Build history of the part. All positions in model axes, mm. Face numbers are marked on the shaded views. Round coordinates to 2 decimals unless told otherwise and drop trailing zeros. Loops run counter-clockwise (first coordinate to the right, second up) from the corner with the lowest first, then second, coordinate; pieces in that order, holes last.
Autodesk Inventor part; units mm, degrees
ref_plane "YZ Plane" through (0, 0, 0) normal (1, 0, 0) x (0, 1, 0)
ref_plane "XZ Plane" through (0, 0, 0) normal (0, 1, 0) x (-1, 0, 0)
ref_plane "XY Plane" through (0, 0, 0) normal (0, 0, 1) x (1, 0, 0)
sketch "Sketch1" plane through (0, 0, 0) normal (1, 0, 0) x (0, 1, 0)
  circle A0 centre (0, 0) radius 4.572
  circle A1 centre (0, 0) radius 8.382
  dimension "d0" = 9.144
  dimension "d1" = 3.81
extrude "Extrusion1" add sketch "Sketch1" along normal blind 19.812
sketch "Sketch2" plane through (0, 0, 0) normal (-1, 0, 0) x (0, 0, 1)
  circle A0 centre (0, 0) radius 8.382
  circle A1 centre (0, 0) radius 7.747
  circle A2 centre (0, 0) radius 8.382
  dimension "d42" = 0
extrude "Extrusion2" add sketch "Sketch2" along normal blind 2.54 contours A0 | A1
sketch "Sketch3" plane through (-2.54, 0, 0) normal (-1, 0, 0) x (0, 0, 1)
  line L0 (19.05, 48.5955) -> (-19.05, 48.5955)
  circle A0 centre (0, 0) radius 8.382
  line L1 (8.382, 0) -> (19.05, 48.5955)
  line L2 (-8.382, 0) -> (-19.05, 48.5955)
  arc A1 (8.382, 0) -> (-8.382, 0) centre (0, 0) ccw
  line L3 (-14.3129, 44.7855) -> (14.3129, 44.7855)
  line L4 (14.3129, 44.7855) -> (6.7152, 10.176)
  arc A2 (6.7152, 10.176) -> (-6.7152, 10.176) centre (0, 0) ccw
  line L5 (-6.7152, 10.176) -> (-14.3129, 44.7855)
  dimension "d6" = 38.1
  dimension "d7" = 19.05
  dimension "d8" = 3.81
extrude "Extrusion3" add sketch "Sketch3" against normal blind 6.35 contours L1 A0 L2 L0
sketch "Sketch6" plane through (-2.54, 44.7855, -14.3129) normal (0, -1, 0) x (1, 0, 0)
  line L0 (6.35, 32.4159) -> (26.9875, 32.4159)
  line L1 (13.4874, 32.4159) -> (13.4874, 26.0989)
  line L2 (26.9875, 32.4159) -> (26.9875, -3.9117)
  point P0 (2.54, 14.3129)
  dimension "d20" = 13.5001
sketch "Sketch10" plane through (0, 0, 0) normal (1, 0, 0) x (0, 0, -1)
  circle A0 centre (0, 0) radius 1.4542
  line L0 (-4.572, 1.4542) -> (4.572, 1.4542)
  line L1 (4.572, 1.4542) -> (4.572, -1.4542)
  line L2 (4.572, -1.4542) -> (-4.572, -1.4542)
  line L3 (-4.572, -1.4542) -> (-4.572, 1.4542)
  circle A1 centre (0, 0) radius 4.572
  dimension "d43" = 0
  dimension "d44" = 0
extrude "Extrusion7" cut sketch "Sketch10" against normal blind 22.225 contours A0 | A0 L0 A1 L2 | A0 L2 A1 L0 | A1 L3 L0 | L0 L1 A1 | A1 L1 L2 | L2 L3 A1
sketch "Sketch13" plane through (-2.54, 48.5955, 19.05) normal (0, 1, 0) x (1, 0, 0)
  line L0 (4.6355, 36.83) -> (1.7145, 36.83)
  line L1 (1.7145, 36.83) -> (1.7145, 33.909)
  line L2 (1.7145, 33.909) -> (4.6355, 33.909)
  line L3 (4.6355, 33.909) -> (4.6355, 36.83)
  line L4 (6.35, 38.1) -> (6.35, 0)
  line L5 (0, 38.1) -> (6.35, 38.1)
  line L6 (4.6228, 4.191) -> (1.7018, 4.191)
  line L7 (1.7018, 4.191) -> (1.7018, 1.27)
  line L8 (1.7018, 1.27) -> (4.6228, 1.27)
  line L9 (4.6228, 1.27) -> (4.6228, 4.191)
  line L10 (0, 0) -> (6.35, 0)
  line L11 (0, 0) -> (0, 38.1)
  line L12 (0, 0) -> (6.35, 0)
  line L13 (6.35, 38.1) -> (6.35, 0)
  line L14 (0, 38.1) -> (6.35, 38.1)
  point P0 (2.54, 19.05)
  dimension "d32" = 2.921
  dimension "d33" = 2.921
  dimension "d34" = 1.7145
  dimension "d35" = 1.27
  dimension "d36" = 2.921
  dimension "d37" = 2.921
  dimension "d38" = 1.7272
  dimension "d39" = 1.27
extrude "Extrusion9" add sketch "Sketch13" along normal blind 3.81 contours L3 L2 L1 L0 | L4 L10 L11 L5 | L9 L8 L7 L6
sketch "Sketch14" plane through (0, 0, 0) normal (-1, 0, 0) x (0, 0, 1)
  arc A0 (4.3346, -1.4542) -> (4.572, 0) centre (0, 0) ccw
  line L0 (4.3346, -1.4542) -> (4.572, -1.4542)
  line L1 (4.572, -1.4542) -> (4.572, 0)
  arc A1 (4.572, 0) -> (4.3346, 1.4542) centre (0, 0) ccw
  line L2 (4.572, 0) -> (4.572, 1.4542)
  line L3 (4.572, 1.4542) -> (4.3346, 1.4542)
  arc A2 (-4.572, 0) -> (-4.3346, -1.4542) centre (0, 0) ccw
  line L4 (-4.572, 0) -> (-4.572, -1.4542)
  line L5 (-4.572, -1.4542) -> (-4.3346, -1.4542)
  arc A3 (-4.3346, 1.4542) -> (-4.572, 0) centre (0, 0) ccw
  line L6 (-4.3346, 1.4542) -> (-4.572, 1.4542)
  line L7 (-4.572, 1.4542) -> (-4.572, 0)
extrude "Extrusion10" add sketch "Sketch14" along normal blind 2.54
sketch "Sketch15" plane through (-2.54, 0, 0) normal (-1, 0, 0) x (0, 0, 1)
  circle A0 centre (0, 0) radius 41.275
  circle A1 centre (0, 0) radius 44.45
  dimension "d47" = 82.55
  dimension "d48" = 88.9
extrude "Extrusion11" add sketch "Sketch15" against normal blind 2.54
sketch "Sketch16" plane through (0, 0, 0) normal (1, 0, 0) x (0, 0, -1)
  circle A0 centre (0, 0) radius 44.45
  circle A1 centre (0, 0) radius 41.275
  dimension "d51" = 82.55
extrude "Extrusion12" add sketch "Sketch16" along normal blind 31.75
sketch "Sketch19" plane through (-2.54, 0, 0) normal (-1, 0, 0) x (0, 0, 1)
  line L0 (4.3346, 1.4542) -> (-4.3346, 1.4542)
  arc A0 (-16.671, 37.7585) -> (16.671, 37.7585) centre (0, 0) ccw
  line L1 (-4.3346, 1.4542) -> (-41.2494, 1.4542)
  line L2 (4.3346, 1.4542) -> (41.2494, 1.4542)
  circle A1 centre (0, 0) radius 8.382
  line L3 (-4.3346, -1.4542) -> (4.3346, -1.4542)
  line L4 (4.3346, 1.4542) -> (-4.3346, 1.4542)
  line L5 (-41.2494, -1.4542) -> (41.2494, -1.4542)
extrude "Extrusion14" add sketch "Sketch19" against normal blind 6.35 contours L2 A1 L5 L3 L1 L0 | L2 A0 L5 A1 | A1 L5 A0 L1
sketch "Sketch20" plane through (3.81, 0, 0) normal (1, 0, 0) x (0, 0, -1)
  arc A0 (4.3346, -1.4542) -> (4.3346, 1.4542) centre (0, 0) ccw
  line L0 (4.3346, 1.4542) -> (-4.3346, 1.4542)
  arc A1 (-4.3346, 1.4542) -> (-4.3346, -1.4542) centre (0, 0) ccw
  line L1 (-4.3346, -1.4542) -> (4.3346, -1.4542)
extrude "Extrusion15" cut sketch "Sketch20" against normal blind 6.35
sketch "Sketch21" plane through (-2.54, 0, 0) normal (-1, 0, 0) x (0, 0, 1)
  arc A0 (-8.2549, -1.4542) -> (8.2549, -1.4542) centre (0, 0) ccw
  line L0 (1.8492, -8.1755) -> (1.8492, -41.2336)
  arc A1 (-41.2494, -1.4542) -> (41.2494, -1.4542) centre (0, 0) ccw
  line L1 (-1.8492, -41.2336) -> (-1.8492, -8.1755)
  arc A2 (-1.8492, -8.1755) -> (1.8492, -8.1755) centre (0, 0) ccw
  arc A3 (-1.8492, -41.2336) -> (1.8492, -41.2336) centre (0, 0) ccw
extrude "Extrusion16" add sketch "Sketch21" against normal blind 6.35
sketch "Sketch23" plane through (3.81, 0, 0) normal (1, 0, 0) x (0, 0, -1)
  line L0 (19.05, 52.4055) -> (-19.05, 52.4055)
  line L1 (-19.05, 48.5955) -> (-19.05, 52.4055)
  line L2 (19.05, 52.4055) -> (-19.05, 52.4055)
  line L3 (-19.05, 52.4055) -> (-19.05, 48.5955)
  line L4 (-19.05, 48.5955) -> (19.05, 48.5955)
  line L5 (19.05, 48.5955) -> (19.05, 52.4055)
  point P0 (0, 0)
extrude "Extrusion17" add sketch "Sketch23" along normal blind 19.05
properties part number "BasicThrustMotorHousing"
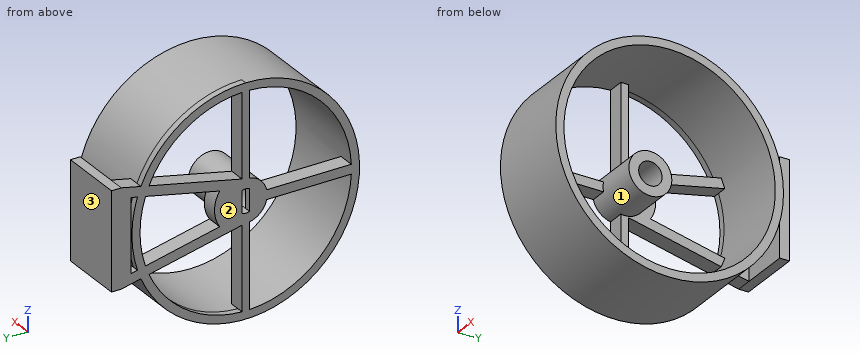
(1) Pull direction Y, two halves, no side cores. Call the marked faces 1, 2 and 3: +Y half, -Y half, draft (parallel to the pull), parting line (faces both ways), or undercut.
Responses:
face 1: undercut
face 2: draft
face 3: +Y half
(2) Slice it at A-A on x = 6. Count the separate pieces of the cut face and the enclosed holes in it, plus the area to 3 significant figures.
Responses:
separate pieces: 3
enclosed holes: 2
area: 1,160 mm2
(3) Slice it at B-B on z = -31. List the corners of the cut face in (x, y), plus the area to 3 significant figures.
Responses:
outline: (-2.54, -31.86) - (31.75, -31.86) - (31.75, -27.25) - (-2.54, -27.25) - close; (-2.54, -1.45) - (3.81, -1.45) - (3.81, 1.45) - (-2.54, 1.45) - close; (-2.54, 27.25) - (31.75, 27.25) - (31.75, 31.86) - (-2.54, 31.86) - close
area: 334 mm2
(4) Pin check, flat tips, straight feed: P1, Ø5, axis at x = 0, z = -23, coming from the -Y side; P2, Ø2, axis at x = 6, z = 27.5, coming from the +Y side; P3, Ø3, axis at x = 2, z = 17, coming from the -Y side; P4, Ø1.5, axis at y = 33.5, z = -17.5, coming from the +X side. Stop position of each tip, or through.
Responses:
P1: stops at y = -39.44
P2: stops at y = 35.69
P3: stops at y = -41.66
P4: passes through
(5) Probe line 1 (Z direction, x = 14, y = 0) (3 decimals); line 2 (Y direction, x = 25, z = 0) (3 decimals); line 3 (Y direction, x = 6, z = -1). List the from-to ranges inside material, lowest first.
Responses:
line 1: z = -44.45 to -41.275, -8.382 to -4.572, 4.572 to 8.382, 41.275 to 44.45
line 2: y = -44.45 to -41.275, 41.275 to 44.45
line 3: y = -44.44 to -41.26, -8.32 to -4.46, 4.46 to 8.32, 41.26 to 44.44, 48.6 to 52.41
